For this review, use the dimensioned drawing (mm, ordinates from the lowest corner) and the shaded views. Give positions to 0.01 mm unless a question says otherwise; leave off trailing zeros. Order: outer loops, then holes, each group sorted by start corner. A loop starts at its lowest first (then second) coordinate and runs counter-clockwise, first axis right, second up.
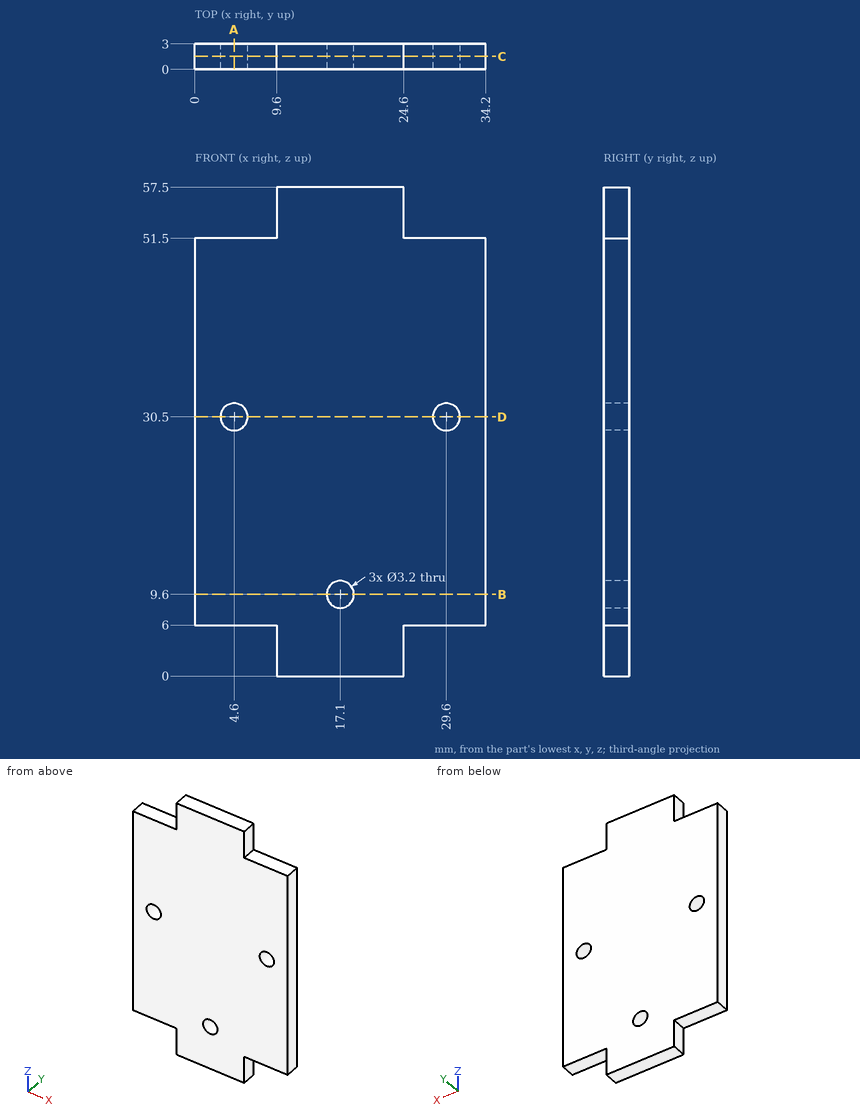
1. Take a section at B-B (z = 9.6). State the section outline as (x, y) points.
Recorded:
outline: (0, 0) - (15.5, 0) - (15.5, 3) - (0, 3) - close; (18.7, 0) - (34.2, 0) - (34.2, 3) - (18.7, 3) - close
2. Take a section at A-A (x = 4.6). State the section outline as (y, z) points, then the cut area to 3 significant figures.
Recorded:
outline: (0, 6) - (3, 6) - (3, 28.9) - (0, 28.9) - close; (0, 32.1) - (3, 32.1) - (3, 51.5) - (0, 51.5) - close
area: 127 mm2
3. Take a section at D-D (z = 30.5). State the section outline as (x, y) points, then the cut area to 3 significant figures.
Recorded:
outline: (0, 0) - (3, 0) - (3, 3) - (0, 3) - close; (6.2, 0) - (28, 0) - (28, 3) - (6.2, 3) - close; (31.2, 0) - (34.2, 0) - (34.2, 3) - (31.2, 3) - close
area: 83.4 mm2
4. For pin 1 (0.9 mm diameter, centred on y = 1.5, z = 53.5, fed in from -X); pin 2 (1.5 mm diameter, centred on x = 29.5, y = 1.5, fed in from +Z); pin 3 (0.9 mm diameter, centred on x = 6.5, y = 2, fed in from -Z), all flat-tipped, find the tip position at first contact; note any pin that passes through.
Recorded:
pin 1: stops at x = 9.6
pin 2: stops at z = 51.5
pin 3: stops at z = 6
5. Take a section at C-C (y = 1.55). State the section outline as (x, z) points, then the cut area to 3 significant figures.
Recorded:
outline: (0, 6) - (9.6, 6) - (9.6, 0) - (24.6, 0) - (24.6, 6) - (34.2, 6) - (34.2, 51.5) - (24.6, 51.5) - (24.6, 57.5) - (9.6, 57.5) - (9.6, 51.5) - (0, 51.5) - close; hole circle Ø3.2 at (4.6, 30.5); hole circle Ø3.2 at (17.1, 9.6); hole circle Ø3.2 at (29.6, 30.5)
area: 1,710 mm2
6. For line 1 along Z through (x, y) = (17.1, 1.25); line 2 along Z through (x, y) = (29.5, 0.65); line 3 along Z through (x, y) = (6.5, 2.8), list the stretches that pass through material, from the lowest coordinate up.
Recorded:
line 1: z = 0 to 8, 11.2 to 57.5
line 2: z = 6 to 28.9, 32.1 to 51.5
line 3: z = 6 to 51.5
